Design review of the part built by this model. Coordinates are the model's own, in mm. Coordinates: 2 decimals unless noted, no trailing zeros. Write each loop counter-clockwise with the first axis right and the second up, starting at its lowest first coordinate (ties: lowest second). Pieces come first, ordered by that corner, then holes. Notation, with made-up numbers: (2, 4) -> (25, 4) arc R17 cw to (25, 29) -> close; hole circle Ø3 at (28, 88.5). An arc over 180 degrees is marked (long way). Answer in a Markdown table with one row per item. Add a question column.
Item 1: To check wall thickness, follow line 1 (Y direction, x = 63, z = 15.5); line 2 (Y direction, x = 14.5, z = 31). State the ranges of each line that lie inside material, in increasing order.
Item 2: Clearance check with flat-ended pins moving along their axes: P1, Ø3, axis at x = 14.5, z = 15, coming from the +Y side; P2, Ø4, axis at x = 42, z = 10, coming from the +Y side; P3, Ø1.5, axis at x = 25, z = 5.5, coming from the +Y side. State where each tip first meets the part, or that it passes through.
Item 3: Take a section at A-A, the plane z = 17. Write out the cut boundary in (x, y), and give its area (3 significant figures).
Item 4: Take a section at B-B, the plane x = 41. Write out the cut boundary in (y, z), and give its area (3 significant figures).
from build123d import *

# Parameters (mm, degrees)
F0_W     = 88.9
F0_H     = 38.1
F1_DEPTH = 1943.1
F3_DEPTH = 38.1
F5_DEPTH = 38.1


with BuildPart() as f1:
    # F0 (on Front) → F1 (new body)
    with BuildSketch(Plane.XZ):
        with Locations((44.45, 19.05)):
            Rectangle(F0_W, F0_H)
    extrude(amount=F1_DEPTH)

    # F2 (on face) → F3 (cut, through all)
    with BuildSketch(Plane.XY.offset(38.1)):
        Polygon((88.9, -1728.476414), (0, -1943.1), (88.9, -1943.1), align=None)
    extrude(amount=-F3_DEPTH, mode=Mode.SUBTRACT)

    # F4 (on face) → F5 (cut, through all)
    with BuildSketch(Plane.XY.offset(38.1)):
        Polygon((88.9, 0), (0, 0), (88.9, -88.9), align=None)
    extrude(amount=-F5_DEPTH, mode=Mode.SUBTRACT)


solid = f1.part
Answers:
| question | item | result |
|---|---|---|
| 1 | line 1 | y = -1791 to -63 |
| 1 | line 2 | y = -1908.09 to -14.5 |
| 2 | P1 | stops at y = -13 |
| 2 | P2 | stops at y = -40 |
| 2 | P3 | stops at y = -24.25 |
| 3 | outline | (0, -1943.1) -> (88.9, -1728.48) -> (88.9, -88.9) -> (0, 0) -> close |
| 3 | area | 159,000 mm^2 |
| 4 | outline | (-1844.12, 0) -> (-41, 0) -> (-41, 38.1) -> (-1844.12, 38.1) -> close |
| 4 | area | 68,700 mm^2 |
